The model under review builds one solid part; all positions refer to its coordinate system, in mm. Face numbers are marked on the shaded views. Coordinates: 2 decimals unless noted, no trailing zeros. Loops run counter-clockwise (first coordinate to the right, second up) from the corner with the lowest first, then second, coordinate; pieces in that order, holes last. Notation, with made-up numbers: M 0,68.25 L 26,68.25 A23 ccw 26,98.25 Z; hole C 71.5,-33 d7. An arc over 180 degrees is marked long. Use CSV: the item, a comma, the result in double quotes. Start each with the question number.
1. Clearance check with flat-ended pins moving along their axes: P1, Ø14, axis at x = 193, y = 1, coming from the +Z side; P2, Ø1, axis at x = 257.5, z = 13, coming from the +Y side; P3, Ø5, axis at x = 88, z = 48.5, coming from the -Y side; P4, Ø12, axis at y = 10.5, z = 23, coming from the +X side. State where each tip first meets the part, or that it passes through.
2. For L1, parallel to Y at x = 0, z = 23 (3 decimals); L2, parallel to Y at x = 178, z = -16.5; L3, parallel to Z at x = 126.5, y = -3, list the stretches that pass through material, from the lowest coordinate up.
3. Add section C-C, the plane z = 59. Write out the cut boundary in (x, y) (3 decimals), then the cut area to 3 significant figures.
4. Add section A-A, the plane x = 0. Write out the cut boundary in (y, z) (3 decimals), then the cut area to 3 significant figures.
5. Add section B-B, the plane y = 0. Write out the cut boundary in (x, z) (3 decimals), then the cut area to 3 significant figures.
6. Add section D-D, the plane y = 15. Write out the cut boundary in (x, z) (3 decimals), then the cut area to 3 significant figures.
7. Draft analysis for pull direction X (two halves, no side actions). For the marked faces 1, 2 and 3, state which applies: +X half, -X half, draft (parallel to the pull), parting line (faces both ways), or undercut.
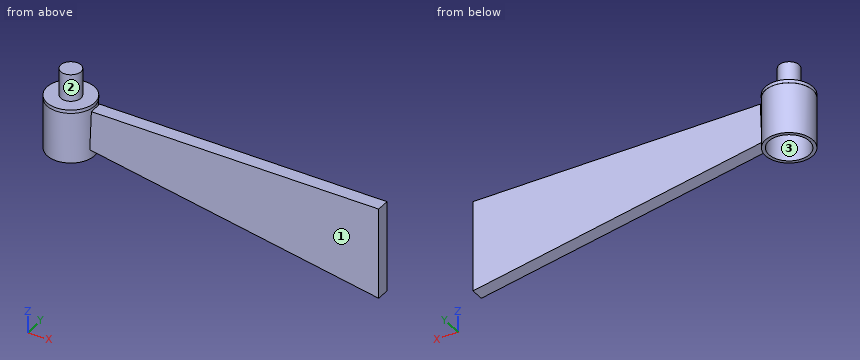
from build123d import *

# Parameters (mm, degrees)
F0_R          = 22.225
F0_R_2        = 19.05
F1_DEPTH      = 47.625
F2_R          = 22.328019
F3_DEPTH      = 3.16947
F4_R          = 9.525
F5_DEPTH      = 25.4
F5_DEPTH_BACK = 25.4
F7_DEPTH      = 6.35
F7_DEPTH_BACK = 6.35


with BuildPart() as f1:
    # F0 (on Top) → F1 (new body)
    with BuildSketch(Plane.XY):
        Circle(F0_R)
        Circle(F0_R_2, mode=Mode.SUBTRACT)
    extrude(amount=F1_DEPTH)

    # F2 (on face) → F3 (join)
    with BuildSketch(Plane.XY.offset(47.625)):
        Circle(F2_R)
    extrude(amount=F3_DEPTH)

    # F4 (on face) → F5 (join, two sides)
    with BuildSketch(Plane.XY.offset(50.79447)) as f5_sk:
        Circle(F4_R)
    extrude(amount=F5_DEPTH)
    extrude(f5_sk.sketch, amount=-F5_DEPTH_BACK)

    # F6 (on Front) → F7 (join, two sides)
    with BuildSketch(Plane.XZ) as f7_sk:
        Polygon((293.185323, 46.228472), (23.211915, 46.228472), (21.699471, 9.1733), (293.185323, -39.225295), align=None)
    extrude(amount=F7_DEPTH)
    extrude(f7_sk.sketch, amount=-F7_DEPTH_BACK)


solid = f1.part
Computed:
1,P1,"stops at z = 46.23"
1,P2,"stops at y = 6.35"
1,P3,"stops at y = -6.35"
1,P4,"stops at x = 293.19"
2,L1,"y = -22.225 to -19.05, 19.05 to 22.225"
2,L2,"y = -6.35 to 6.35"
2,L3,"z = -9.51 to 46.23"
3,outline,"C 0,0 d19.05"
3,area,"285 mm^2"
4,outline,"M -22.328,47.625 L -22.225,47.625 L -22.225,0 L -19.05,0 L -19.05,47.625 L -9.525,47.625 L -9.525,25.394 L 9.525,25.394 L 9.525,47.625 L 19.05,47.625 L 19.05,0 L 22.225,0 L 22.225,47.625 L 22.328,47.625 L 22.328,50.794 L 9.525,50.794 L 9.525,76.194 L -9.525,76.194 L -9.525,50.794 L -22.328,50.794 Z"
4,area,"1,350 mm^2"
5,outline,"M -22.328,47.625 L -22.225,47.625 L -22.225,0 L -19.05,0 L -19.05,47.625 L -9.525,47.625 L -9.525,25.394 L 9.525,25.394 L 9.525,47.625 L 19.05,47.625 L 19.05,0 L 22.225,0 L 22.225,9.08 L 293.185,-39.225 L 293.185,46.228 L 23.212,46.228 L 22.225,22.049 L 22.225,47.625 L 22.328,47.625 L 22.328,50.794 L 9.525,50.794 L 9.525,76.194 L -9.525,76.194 L -9.525,50.794 L -22.328,50.794 Z"
5,area,"17,900 mm^2"
6,outline,"M -16.539,47.625 L -16.4,47.625 L -16.4,0 L -11.743,0 L -11.743,47.625 L 11.743,47.625 L 11.743,0 L 16.4,0 L 16.4,47.625 L 16.539,47.625 L 16.539,50.794 L -16.539,50.794 Z"
6,area,"548 mm^2"
7,face 1,"draft"
7,face 2,"parting line"
7,face 3,"undercut"
